Design review of the part built by this model. Coordinates are the model's own, in mm. Face numbers are marked on the shaded views. A direction names the side the tool comes from. Coordinates: 2 decimals unless noted, no trailing zeros. Put each result on its own line as item: value. Start each with the question number.
(1) Clearance check with flat-ended pins moving along their axes: pin 1 (5 mm diameter, centred on y = 5, z = 38, fed in from +X); pin 2 (5 mm diameter, centred on x = -6, y = 1.5, fed in from +Z); pin 3 (2 mm diameter, centred on y = 3, z = 21.5, fed in from -X); pin 4 (9.5 mm diameter, centred on x = 0, z = 39.28, fed in from +Y). State where each tip first meets the part, or that it passes through.
(2) The part is to be moulded in two halves that separate along X. For the marked faces 3 and 4, say which applies: +X half, -X half, draft (parallel to the pull), parting line (faces both ways), or undercut.
(3) For probe 1 along Y at (x, z) = (-7, 30.5); probe 2 along X at (y, z) = (11.5, 41); probe 3 along Z at (x, y) = (9, 8.25), list the stretches that pass through material, from the lowest coordinate up. Write a range as [from, to].
(4) For the marked faces 1 and 2, list the 3-axis set-ups (+Z, -Z, +X, -X, +Y, -Y) from which the entire face can be reached by the end or side of a thin tool; tool diameter is ignored.
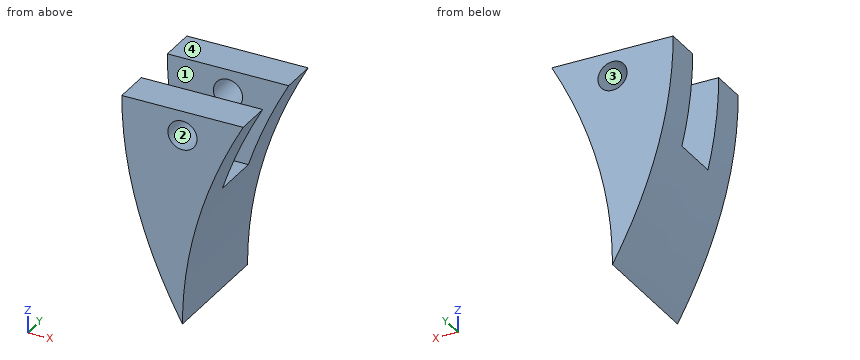
```python
from build123d import *

# Parameters (mm, degrees)
SKETCH_1_W          = 25
SKETCH_1_H          = 25
EXTRUDE_1_DEPTH     = 44.284173786
SKETCH_2_R          = 3
CUT_EXTRUDE_1_DEPTH = 36.344532851
SKETCH_4_W          = 25
SKETCH_4_H          = 10
CUT_EXTRUDE_2_DEPTH = 18.639834826
CUT_EXTRUDE_4_DEPTH = 30


with BuildPart() as part:
    # 스케치1 → 보스-돌출1 (new body)
    with BuildSketch(Plane.XY):
        Rectangle(SKETCH_1_W, SKETCH_1_H)
    extrude(amount=EXTRUDE_1_DEPTH)

    # 스케치2 → 컷-돌출1 (cut)
    with BuildSketch(Plane(origin=(0, 12.5, 0), x_dir=(1, 0, 0), z_dir=(0, 1, 0))):
        with Locations(Location((0, -39.284173786, 0), (0, 0, 270))):
            Circle(SKETCH_2_R)
    extrude(amount=-CUT_EXTRUDE_1_DEPTH, mode=Mode.SUBTRACT)

    # 스케치4 → 컷-돌출2 (cut)
    with BuildSketch(Plane.XY.offset(44.284173786)):
        Rectangle(SKETCH_4_W, SKETCH_4_H)
    extrude(amount=-CUT_EXTRUDE_2_DEPTH, mode=Mode.SUBTRACT)

    # 스케치5 → 컷-돌출4 (cut)
    with BuildSketch(Plane(origin=(0, 12.5, 0), x_dir=(1, 0, 0), z_dir=(0, 1, 0))):
        with BuildLine():
            add(Edge.make_bspline(
                [(0, 0), (-0.013056864, -22.058961494), (12.5, -44.284173786)],
                knots=[0, 0, 0, 1, 1, 1], degree=2))
            Line((12.5, -44.284173786), (12.5, 0))
            Line((12.5, 0), (0, 0))
        make_face()
        with BuildLine():
            add(Edge.make_bspline(
                [(0, 0), (-12.5, -22.142086893), (-12.5, -44.284173786)],
                knots=[0, 0, 0, 1, 1, 1], degree=2))
            Line((0, 0), (-12.5, 0))
            Line((-12.5, 0), (-12.5, -44.284173786))
        make_face()
    extrude(amount=-CUT_EXTRUDE_4_DEPTH, mode=Mode.SUBTRACT)


solid = part.part
```
Computed values:
1. pin 1: stops at x = 10.46
1. pin 2: stops at z = 25.64
1. pin 3: stops at x = -9.48
1. pin 4: stops at y = 12.5
2. face 3: undercut
2. face 4: draft
3. probe 1: y = [-12.5, -5], [5, 12.5]
3. probe 2: x = [-12.43, -2.46], [2.46, 10.72]
3. probe 3: z = [37.56, 44.28]
4. face 1: +Z, +X, -X
4. face 2: +Y, -Y
